```python
from build123d import *

# Parameters (mm, degrees)
SKETCH1_R                = 30
BOSS_EXTRUDE1_DEPTH      = 120
SKETCH2_R                = 50
BOSS_EXTRUDE2_DEPTH      = 40
BOSS_EXTRUDE2_DEPTH_BACK = 20
SKETCH3_R                = 20
BOSS_EXTRUDE3_DEPTH      = 300


with BuildPart() as part:
    # Sketch1 → Boss-Extrude1 (new body)
    with BuildSketch(Plane.XY):
        Circle(SKETCH1_R)
    extrude(amount=BOSS_EXTRUDE1_DEPTH)

    # Sketch2 → Boss-Extrude2 (add, two sides)
    with BuildSketch(Plane(origin=(0, 0, 0), x_dir=(-1, 0, 0), z_dir=(0, 0.984807753, -0.173648178))) as boss_extrude2_sk:
        Circle(SKETCH2_R)
    extrude(amount=BOSS_EXTRUDE2_DEPTH)
    extrude(boss_extrude2_sk.sketch, amount=-BOSS_EXTRUDE2_DEPTH_BACK)

    # Sketch3 → Boss-Extrude3 (add)
    with BuildSketch(Plane(origin=(0, 39.39231012, -6.945927107), x_dir=(1, 0, 0), z_dir=(0, 0.984807753, -0.173648178))):
        Circle(SKETCH3_R)
    extrude(amount=BOSS_EXTRUDE3_DEPTH)


solid = part.part
```
Can you work these out from the model? Positions are in its coordinate system, mm. A direction names the side the tool comes from. Coordinates: 2 decimals unless noted, no trailing zeros. Loops run counter-clockwise (first coordinate to the right, second up) from the corner with the lowest first, then second, coordinate; pieces in that order, holes last. Notation, with made-up numbers: (54, -30.5) - (64, -30.5) arc R31 ccw to (64, 6.5) - close; hole circle Ø3 at (33.25, 83). An arc over 180 degrees is marked (long way). Use a Markdown table: item, result.
Item 1: Will these pins go through, and if not, where does the flat tip stop? pin 1 (3 mm diameter, centred on x = -19.5, y = 128, fed in from -Z); pin 2 (6 mm diameter, centred on x = -10.5, z = -46.5, fed in from -Y); pin 3 (10.5 mm diameter, centred on x = -2.5, y = -23.5, fed in from -Z).
Numbers:
| item | result |
|---|---|
| pin 1 | stops at z = -31.43 |
| pin 2 | stops at y = -28.27 |
| pin 3 | stops at z = -47.51 |
Item 2: I want a section at A-A on z = 96.5. Please give me the cut outline in (x, y), and give its area (3 significant figures).
Numbers:
| item | result |
|---|---|
| outline | circle Ø60 at (0, 0) |
| area | 2,830 mm2 |
Item 3: We'd pull the mould along Y, two halves only. Please class faces 1 (the face through (0.7, 35.655, -28.141)), 2 (the face through (0.7, -22.06, -9.94)), 3 (the face through (-0.28, 334.786, -59.316)): released by +Y, released by -Y, zero draft, split by the parting line, or undercut.
Numbers:
| item | result |
|---|---|
| face 1 | undercut |
| face 2 | released by -Y |
| face 3 | released by +Y |
Item 4: For faces 4 (the face through (-6.503, -29.287, 72.493)), 5 (the face through (10.8, 182.1, -49.2)), which set-ups out of +Z, -Z, +X, -X, +Y, -Y let a thin tool reach every point of the face, with its end or its side?
Numbers:
| item | result |
|---|---|
| face 4 | +Z |
| face 5 | none |
Item 5: If I drill on probe 1 along Y at (x, z) = (11, 83); probe 2 along X at (y, z) = (-7, 98.5); probe 3 along Y at (x, z) = (-22.5, 71), over which ranges is the centre line in solid material (lowest first)? Write a range as from..to.
Numbers:
| item | result |
|---|---|
| probe 1 | y = -27.91..27.91 |
| probe 2 | x = -29.17..29.17 |
| probe 3 | y = -19.84..19.84 |
Item 6: I want a section at C-C on x = -36. Please give me the cut outline in (y, z).
Numbers:
| item | result |
|---|---|
| outline | (-25.72, -30.7) - (33.37, -41.12) - (45.42, 27.23) - (-13.67, 37.64) - close |
Item 7: I want a section at B-B on x = -10. Please give me the cut outline in (y, z).
Numbers:
| item | result |
|---|---|
| outline | (-28.28, 0) - (-20.31, 0) - (-28.2, -44.77) - (30.89, -55.19) - (36.38, -24) - (331.83, -76.1) - (337.84, -41.98) - (42.4, 10.11) - (47.9, 41.3) - (28.28, 44.76) - (28.28, 120) - (-28.28, 120) - close |
